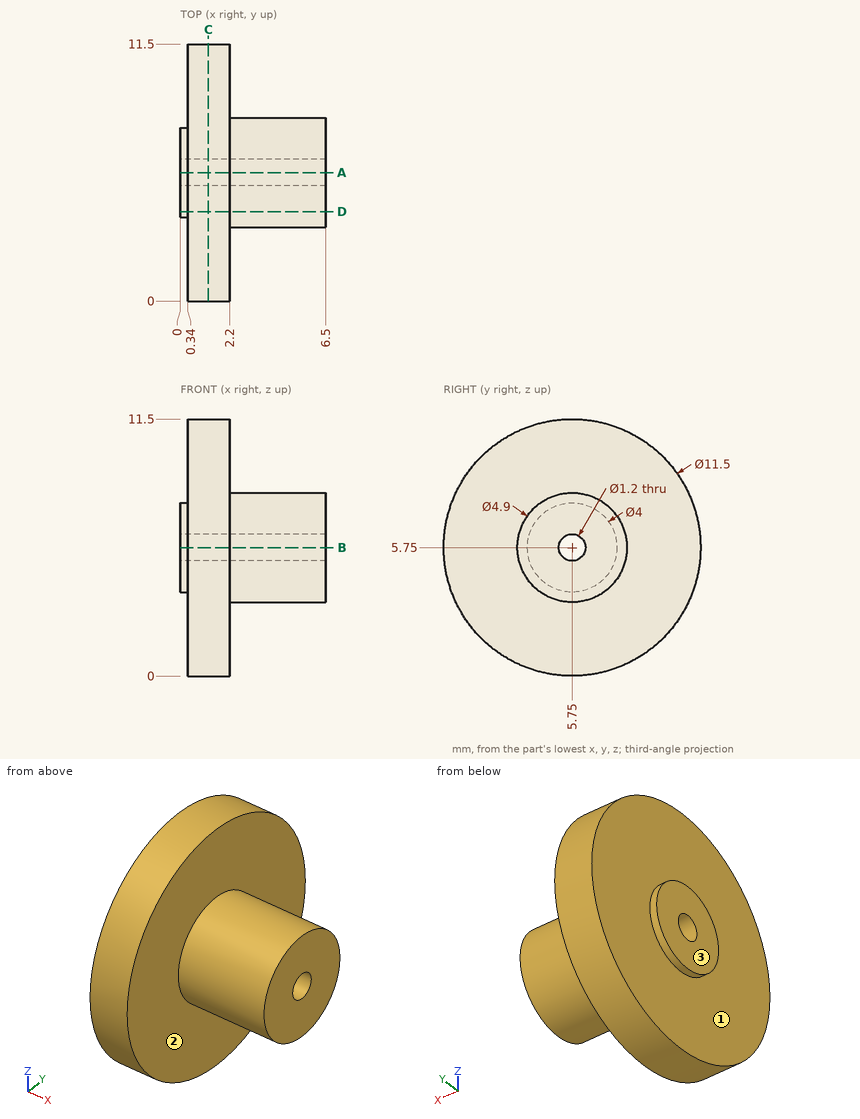
Input: dimensioned drawing with shaded views. Units: mm. Origin: part minimum x, y, z. A direction names the side the tool comes from. Coordinates: 2 decimals unless noted, no trailing zeros. Loops run counter-clockwise (first coordinate to the right, second up) from the corner with the lowest first, then second, coordinate; pieces in that order, holes last. Notation, with made-up numbers: M 26,-9.5 L 53,-9.5 A10 ccw 53,-4.5 Z; hole C -33,82.5 d9. An arc over 180 degrees is marked long. Use a Markdown table: item, result. Add a question column.
Q1. Material intervals for L1, parallel to Z at x = 3.75, y = 5.75; L2, parallel to X at y = 11, z = 7, sorted ascending.
Q2. Section query D-D, the plane y = 4. Return loops of the section in (x, z).
Q3. Access query for the marked faces 1, 2 and 3. Directions: +Z, -Z, +X, -X, +Y, -Y. A direction counts if a zero-diameter tool reaches every point of the face in a straight line with its end or side. Return the directions, or none.
Q4. Section query C-C, the plane x = 1.25. Return loops of the section in (y, z).
Q5. First-contact query: pin 1 (1 mm diameter, centred on x = 2, z = 8, fed in from -Y); pin 2 (2 mm diameter, centred on x = 4.5, y = 2.5, fed in from -Z); pin 3 (1 mm diameter, centred on y = 1, z = 6, fed in from +X). Flat tips, straight axial feed; report the tip coordinate or a pass-through.
Q6. Section query A-A, the plane y = 5.75. Return loops of the section in (x, z).
Result:
| question | item | result |
|---|---|---|
| 1 | L1 | z = 3.3 to 5.15, 6.35 to 8.2 |
| 1 | L2 | x = 0.34 to 2.2 |
| 2 | outline | M 0,4.78 L 0.34,4.78 L 0.34,0.27 L 2.2,0.27 L 2.2,4.04 L 6.5,4.04 L 6.5,7.46 L 2.2,7.46 L 2.2,11.23 L 0.34,11.23 L 0.34,6.72 L 0,6.72 Z |
| 3 | face 1 | -X |
| 3 | face 2 | +X |
| 3 | face 3 | +Z, -Z, -X, +Y, -Y |
| 4 | outline | C 5.75,5.75 d11.5; hole C 5.75,5.75 d1.2 |
| 5 | pin 1 | stops at y = 0.27 |
| 5 | pin 2 | stops at z = 4.78 |
| 5 | pin 3 | stops at x = 2.2 |
| 6 | outline | M 0,3.75 L 0.34,3.75 L 0.34,0 L 2.2,0 L 2.2,3.3 L 6.5,3.3 L 6.5,5.15 L 0,5.15 Z; M 0,6.35 L 6.5,6.35 L 6.5,8.2 L 2.2,8.2 L 2.2,11.5 L 0.34,11.5 L 0.34,7.75 L 0,7.75 Z |
